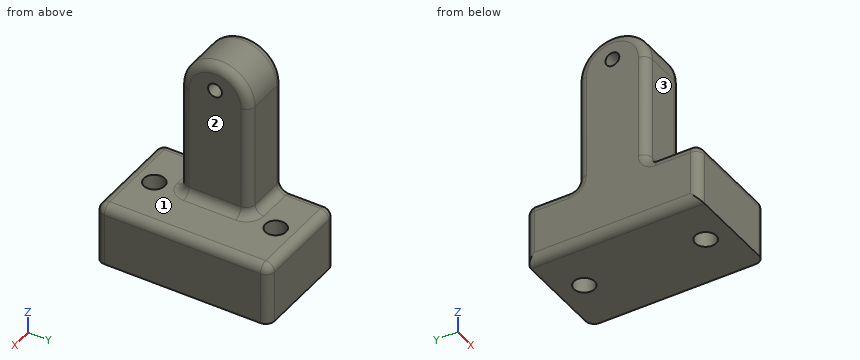
from build123d import *

# Parameters (mm, degrees)
F0_W     = 60
F0_H     = 100
F1_DEPTH = 100
F2_R     = 6
F3_DEPTH = 100
F4_R     = 6
F5_DEPTH = 65
F6_W     = 30
F6_H     = 20
F7_ANGLE = 180
F8_R     = 4
F9_DEPTH = 50
F10_R    = 5


with BuildPart() as f1:
    # F0 (on Top) → F1 (new body)
    with BuildSketch(Plane.XY):
        Rectangle(F0_W, F0_H)
    extrude(amount=F1_DEPTH)

    # F2 (on face) → F3 (cut)
    with BuildSketch(Plane.XY.offset(100)):
        with Locations((0, 35)):
            Circle(F2_R)
        with Locations((0, -35)):
            Circle(F2_R)
    extrude(amount=-F3_DEPTH, mode=Mode.SUBTRACT)

    # F4 (on face) → F5 (cut)
    with BuildSketch(Plane.XY.offset(100)):
        Polygon((0, 20), (0, 0), (0, -20), (-30, -20), (-30, -50), (30, -50), (30, 50), (-30, 50), (-30, 20), align=None)
        with Locations((0, -35)):
            Circle(F4_R, mode=Mode.SUBTRACT)
        with Locations((0, 35)):
            Circle(F4_R, mode=Mode.SUBTRACT)
    extrude(amount=-F5_DEPTH, mode=Mode.SUBTRACT)

    # F6 (on face) → F7 (revolve)
    with BuildSketch(Plane.XY.offset(100)):
        with Locations((-15, -10)):
            Rectangle(F6_W, F6_H)
    revolve(axis=Axis((-15, 0, 100), (-1, 0, 0)), revolution_arc=F7_ANGLE)

    # F8 (on face) → F9 (cut)
    with BuildSketch(Plane(origin=(-30, 0, 0), x_dir=(0, -1, 0), z_dir=(-1, 0, 0))):
        with Locations((0, 105)):
            Circle(F8_R)
    extrude(amount=-F9_DEPTH, mode=Mode.SUBTRACT)

    # F10
    f10_edges = [f1.edges().sort_by_distance(p)[0] for p in [
        (-30, 20, 67.5),
        (-30, 35, 35),
        (-30, 50, 17.5),
        (-30, 0, 0),
        (-30, -35, 35),
        (-30, -50, 17.5),
        (0, -50, 35),
        (30, -50, 17.5),
        (30, 0, 35),
        (-15, -20, 35),
        (0, -20, 67.5),
        (30, 50, 17.5),
        (0, 50, 35),
        (0, 0, 35),
        (-15, 20, 35),
        (-30, -20, 67.5),
        (-30, 0, 120),
        (0, 20, 67.5),
        (0, 0, 120),
    ]]
    fillet(f10_edges, radius=F10_R)


solid = f1.part
Source: CAD feature listing. Evaluate the final solid. Frame: model axes, mm. Face numbers are marked on the shaded views. A direction names the side the tool comes from. Round coordinates to 2 decimals unless told otherwise and drop trailing zeros. Loops run counter-clockwise (first coordinate to the right, second up) from the corner with the lowest first, then second, coordinate; pieces in that order, holes last.
Q1. Ray query, line 1 (Y direction, x = 0, z = 22); line 2 (Z direction, x = -5, y = -29.5); line 3 (X direction, y = -10.5, z = 43). Return the intervals inside material, ascending.
Q2. First-contact query: P1, Ø13, axis at y = 0, z = 105, coming from the +X side; P2, Ø6, axis at x = -12.5, z = 66, coming from the -Y side; P3, Ø1.5, axis at x = 22.5, y = 39.5, coming from the +Z side. Flat tips, straight axial feed; report the tip coordinate or a pass-through.
Q3. Section B-B, the plane x = -23. Return loops of the section in (y, z).
Q4. Section C-C, the plane z = 25.5. Return loops of the section in (x, y), plus the area to 3 significant figures.
Q5. Section A-A, the plane y = 0. Return loops of the section in (x, z), plus the area to 3 significant figures.
Q6. Access query for the marked faces 1, 2 and 3. Directions: +Z, -Z, +X, -X, +Y, -Y. A direction counts if a zero-diameter tool reaches every point of the face in a straight line with its end or side. Return the directions, or none.
Q7. Section D-D, the plane z = 58. Return loops of the section in (x, y).
Solutions:
1. line 1: y = -50 to -41, -29 to 29, 41 to 50
1. line 2: z = 0 to 35
1. line 3: x = -30 to 0
2. P1: stops at x = 0
2. P2: stops at y = -20
2. P3: stops at z = 35
3. outline: (-50, 0) - (50, 0) - (50, 30) arc R5 ccw to (45, 35) - (25, 35) arc R5 cw to (20, 40) - (20, 100) arc R20 ccw to (-20, 100) - (-20, 40) arc R5 cw to (-25, 35) - (-45, 35) arc R5 ccw to (-50, 30) - close; hole circle Ø8 at (0, 105)
4. outline: (-30, -45) arc R5 ccw to (-25, -50) - (25, -50) arc R5 ccw to (30, -45) - (30, 45) arc R5 ccw to (25, 50) - (-25, 50) arc R5 ccw to (-30, 45) - close; hole circle Ø12 at (0, -35); hole circle Ø12 at (0, 35)
4. area: 5,750 mm2
5. outline: (-30, 5) arc R5 ccw to (-25, 0) - (30, 0) - (30, 30) arc R5 ccw to (25, 35) - (5, 35) arc R5 cw to (0, 40) - (0, 101) - (-30, 101) - close; (-30, 109) - (0, 109) - (0, 115) arc R5 ccw to (-5, 120) - (-25, 120) arc R5 ccw to (-30, 115) - close
5. area: 4,390 mm2
6. face 1: +Z, +X
6. face 2: +Z, +X, +Y, -Y
6. face 3: +Z, +X, -X, -Y
7. outline: (-30, -15) arc R5 ccw to (-25, -20) - (-5, -20) arc R5 ccw to (0, -15) - (0, 15) arc R5 ccw to (-5, 20) - (-25, 20) arc R5 ccw to (-30, 15) - close
